Can you work these out from the model? Positions are in its coordinate system, mm. A direction names the side the tool comes from. Coordinates: 2 decimals unless noted, no trailing zeros. Write each loop counter-clockwise with the first axis right and the second up, starting at its lowest first coordinate (ties: lowest second). Pieces come first, ordered by that corner, then holes. Notation, with made-up numbers: (25.25, 19.25) - (75.25, 19.25) arc R20 cw to (75.25, 27.25) - close; hole circle Ø7 at (-4.5, 62.25). An arc over 180 degrees is marked (long way). Use one line per item in the form item = value. Start each with the question number.
(1) Thinking about a two-plate mould opening in X: for faces 4 (the face through (-119, -23, 25)), 5 (the face through (-115, 28, 29)), 6 (the face through (-1.08, -4.88, 4.93)), which applies, pulls with the +X half, pulls with the -X half, needs draft (parallel to the pull), parting line crosses it, or undercut?
(2) If we section it at A-A on z = 36: Please give me the cut outline in (x, y).
(3) On a 3-axis mill with a long thin cutter (end or side, diameter ignored), from which of +Z, -Z, +X, -X, +Y, -Y can I reach the whole of each face in a straight line? I mean faces 1 (the face through (-139, 0, 26.5)), 2 (the face through (-134, 0, 21)), 3 (the face through (32.99, -0.73, 4.93)). Say none if no direction works.
(4) For pin 1 Ø6 at (y, z) = (26, 38.5) entering from +X; pin 2 Ø2 at (x, y) = (-7.5, -20) entering from +Z; pin 3 Ø8 at (x, z) = (-66, 16) entering from +Y; pin 4 Ø8 at (x, y) = (-141.5, -1.5) entering from +Z, each with a flat end and sliding along its axis, tell me the tip position at first contact or that it passes through.
(5) If we section it at C-C on z = 12: Please give me the cut outline in (x, y).
(6) If I drill on probe 1 along Z at (x, y) = (6, -25); probe 2 along X at (y, z) = (13, 21.5), over which ranges is the centre line in solid material (lowest first)? Write a range as from..to.
(7) If we section it at B-B on y = 0: Please give me the cut outline in (x, z), then the cut area to 3 significant figures.
(8) If we section it at D-D on y = -9: Please give me the cut outline in (x, z), then the cut area to 3 significant figures.
```python
from build123d import *

# Parameters (mm, degrees)
SKETCH1_R           = 5
BOSS_EXTRUDE1_DEPTH = 10
SKETCH3_W           = 43
SKETCH3_H           = 43
BOSS_EXTRUDE3_DEPTH = 10
BOSS_EXTRUDE4_DEPTH = 10


with BuildPart() as part:
    # Sketch1 → Boss-Extrude1 (new body)
    with BuildSketch(Plane.XY):
        with BuildLine():
            Line((0, 33), (-144, 33))
            Line((-144, 33), (-144, -33))
            Line((-144, -33), (0, -33))
            ThreePointArc((0, -33), (33, 0), (0, 33))
        make_face()
        Circle(SKETCH1_R, mode=Mode.SUBTRACT)
    extrude(amount=BOSS_EXTRUDE1_DEPTH)

    # Sketch3 → Boss-Extrude3 (add)
    with BuildSketch(Plane.ZY.offset(144)):
        with BuildLine():
            Line((48, 33), (10, 33))
            Line((10, 33), (10, -33))
            Line((10, -33), (48, -33))
            ThreePointArc((48, -33), (81, 0), (48, 33))
        make_face()
        with Locations((48, 0)):
            Rectangle(SKETCH3_W, SKETCH3_H, mode=Mode.SUBTRACT)
    extrude(amount=-BOSS_EXTRUDE3_DEPTH)

    # Sketch4 → Boss-Extrude4 (add)
    with BuildSketch(Plane(origin=(0, 33, 0), x_dir=(1, 0, 0), z_dir=(0, 1, 0))):
        Polygon((-134, -48), (-96, -10), (-134, -10), align=None)
    boss_extrude4 = extrude(amount=-BOSS_EXTRUDE4_DEPTH)

    # Mirror1: Boss-Extrude4 across plane
    add(boss_extrude4.mirror(Plane.ZX))


solid = part.part
```
Reported:
q1.face_4 = needs draft
q1.face_5 = pulls with the +X half
q1.face_6 = undercut
q2.outline = (-144, -33) - (-122, -33) - (-122, -23) - (-134, -23) - (-134, -21.5) - (-144, -21.5) - close; (-144, 21.5) - (-134, 21.5) - (-134, 23) - (-122, 23) - (-122, 33) - (-144, 33) - close
q3.face_1 = +X, -X
q3.face_2 = +Z, +X
q3.face_3 = +Z, -Z, +X
q4.pin_1 = -121.5
q4.pin_2 = 10
q4.pin_3 = through
q4.pin_4 = 81
q5.outline = (-144, -33) - (-98, -33) - (-98, -23) - (-134, -23) - (-134, 23) - (-98, 23) - (-98, 33) - (-144, 33) - close
q6.probe_1 = 0..10
q6.probe_2 = -144..-134
q7.outline = (-144, 0) - (-5, 0) - (-5, 10) - (-134, 10) - (-134, 26.5) - (-144, 26.5) - close; (-144, 69.5) - (-134, 69.5) - (-134, 81) - (-144, 81) - close; (5, 0) - (33, 0) - (33, 10) - (5, 10) - close
q7.area = 1,950 mm2
q8.outline = (-144, 0) - (31.75, 0) - (31.75, 10) - (-134, 10) - (-134, 26.5) - (-144, 26.5) - close; (-144, 69.5) - (-134, 69.5) - (-134, 79.75) - (-144, 79.75) - close
q8.area = 2,020 mm2
